```python
from build123d import *

# Parameters (mm, degrees)
F1_DEPTH = 1.524
F3_DEPTH = 2.54
F4_DEPTH = 3.81
F4_TAPER = 10
F5_W     = 16.791988407
F5_H     = 42.191988407
F6_DEPTH = 6.35


with BuildPart() as f1:
    # F0 (on Top) → F1 (new body)
    with BuildSketch(Plane.XY):
        with BuildLine():
            ThreePointArc((0, 3.175), (0.9299359697, 0.9299359697), (3.175, 0))
            Line((3.175, 0), (22.225, 0))
            ThreePointArc((22.225, 0), (24.4700640303, 0.9299359697), (25.4, 3.175))
            Line((25.4, 3.175), (25.4, 47.625))
            ThreePointArc((25.4, 47.625), (24.4700640303, 49.8700640303), (22.225, 50.8))
            Line((22.225, 50.8), (3.175, 50.8))
            ThreePointArc((3.175, 50.8), (0.9299359697, 49.8700640303), (0, 47.625))
            Line((0, 47.625), (0, 3.175))
        make_face()
    extrude(amount=F1_DEPTH)

    # F2 (on face) → F3 (join)
    with BuildSketch(Plane.XY.offset(1.524)):
        with BuildLine():
            Line((23.7998, 3.175), (23.7998, 47.625))
            ThreePointArc((23.7998, 47.625), (23.338551759, 48.738551759), (22.225, 49.1998))
            Line((22.225, 49.1998), (3.175, 49.1998))
            ThreePointArc((3.175, 49.1998), (2.061448241, 48.738551759), (1.6002, 47.625))
            Line((1.6002, 47.625), (1.6002, 3.175))
            ThreePointArc((1.6002, 3.175), (2.061448241, 2.061448241), (3.175, 1.6002))
            Line((3.175, 1.6002), (22.225, 1.6002))
            ThreePointArc((22.225, 1.6002), (23.338551759, 2.061448241), (23.7998, 3.175))
        make_face()
    extrude(amount=F3_DEPTH)

    # F3_face (on face) → F4 (join)
    with BuildSketch(Plane(origin=(12.7, 25.4, 4.064), x_dir=(1, 0, 0), z_dir=(0, 0, 1))):
        with BuildLine():
            ThreePointArc((9.525, -23.7998), (10.638551759, -23.338551759), (11.0998, -22.225))
            Line((11.0998, -22.225), (11.0998, 22.225))
            ThreePointArc((11.0998, 22.225), (10.638551759, 23.338551759), (9.525, 23.7998))
            Line((9.525, 23.7998), (-9.525, 23.7998))
            ThreePointArc((-9.525, 23.7998), (-10.638551759, 23.338551759), (-11.0998, 22.225))
            Line((-11.0998, 22.225), (-11.0998, -22.225))
            ThreePointArc((-11.0998, -22.225), (-10.638551759, -23.338551759), (-9.525, -23.7998))
            Line((-9.525, -23.7998), (9.525, -23.7998))
        make_face()
    extrude(amount=F4_DEPTH, taper=F4_TAPER)

    # F5 (on face) → F6 (cut)
    with BuildSketch(Plane.XY.offset(7.874)):
        with Locations((12.7, 25.4)):
            Rectangle(F5_W, F5_H)
    extrude(amount=-F6_DEPTH, mode=Mode.SUBTRACT)


solid = f1.part
```
The model under review builds one solid part; all positions refer to its coordinate system, in mm. A direction names the side the tool comes from. Round coordinates to 2 decimals unless told otherwise and drop trailing zeros. Loops run counter-clockwise (first coordinate to the right, second up) from the corner with the lowest first, then second, coordinate; pieces in that order, holes last. Notation, with made-up numbers: (26.5, 19) - (42.5, 19) arc R18 cw to (42.5, 23) - close; hole circle Ø3 at (24.5, 79.25). An arc over 180 degrees is marked (long way). Write each question's results on one line, items separated by ' | '. Start each with the question number.
Q1. Take a section at A-A on z = 3. Give the boundary of the cut face in (x, y) (3 decimals), plus the area to 3 significant figures.
Q2. Take a section at B-B on x = 7. Give the boundary of the cut face in (y, z).
Q3. Draft analysis for pull direction Y (two halves, no side actions). For faces 5 (the flat face through (21.096, 25, 5)), 6 (the flat face through (4.304, 25, 5)), 7 (the conical face through (2.293, 2.312, 5.996)), 8 (the flat face through (1.93, 25.09, 5.94)), state which applies: pulls with the +Y half, pulls with the -Y half, needs draft (parallel to the pull), parting line crosses it, or undercut.
Q4. Take a section at C-C on y = 6. Give the boundary of the cut face in (x, z).
Q5. Take a section at D-D on z = 6.25. Give the boundary of the cut face in (x, y) (3 decimals), plus the area to 3 significant figures.
Q6. Wall thickness on line 1 along X through (y, z) = (33, 2.75); line 2 along Y through (x, z) = (15.75, 1.75); line 3 along X through (y, z) = (20, 5.25): over which ranges is each line inside the solid? List them lowest first. Write a range as [from, to].
Q7. Insertion check: P1, Ø0.8, axis at x = 8, z = 2.5, coming from the +Y side; P2, Ø7.5, axis at x = 16, y = 24, coming from the +Z side; P3, Ø1.9, axis at x = 9, z = 5, coming from the -Y side. Each pin has a flat end and moves straight along its axis. Give the tip position at first contact, or say it passes through.
Q8. Tool access review of faces 1 (the flat face through (13, 49.2, 3)), 2 (the cylindrical face through (23.326, 2.049, 2.776)), 3 (the cylindrical face through (2.074, 48.751, 2.776)), 4 (the flat face through (13, 46.496, 5)): name each direction out of +Z, -Z, +X, -X, +Y, -Y from which nothing blocks a thin tool from reaching the whole face with its end or side.
Data:
1) outline: (1.6, 3.175) arc R1.575 ccw to (3.175, 1.6) - (22.225, 1.6) arc R1.575 ccw to (23.8, 3.175) - (23.8, 47.625) arc R1.575 ccw to (22.225, 49.2) - (3.175, 49.2) arc R1.575 ccw to (1.6, 47.625) - close; hole (4.304, 4.304) - (21.096, 4.304) - (21.096, 46.496) - (4.304, 46.496) - close | area: 346 mm²
2) outline: (0, 0) - (50.8, 0) - (50.8, 1.52) - (49.2, 1.52) - (49.2, 4.06) - (48.53, 7.87) - (46.5, 7.87) - (46.5, 1.52) - (4.3, 1.52) - (4.3, 7.87) - (2.27, 7.87) - (1.6, 4.06) - (1.6, 1.52) - (0, 1.52) - close
3) face 5: undercut | face 6: undercut | face 7: pulls with the -Y half | face 8: needs draft
4) outline: (0, 0) - (25.4, 0) - (25.4, 1.52) - (23.8, 1.52) - (23.8, 4.06) - (23.13, 7.87) - (21.1, 7.87) - (21.1, 1.52) - (4.3, 1.52) - (4.3, 7.87) - (2.27, 7.87) - (1.6, 4.06) - (1.6, 1.52) - (0, 1.52) - close
5) outline: (1.986, 3.175) arc R1.189 ccw to (3.175, 1.986) - (22.225, 1.986) arc R1.189 ccw to (23.414, 3.175) - (23.414, 47.625) arc R1.189 ccw to (22.225, 48.814) - (3.175, 48.814) arc R1.189 ccw to (1.986, 47.625) - close; hole (4.304, 4.304) - (21.096, 4.304) - (21.096, 46.496) - (4.304, 46.496) - close | area: 294 mm²
6) line 1: x = [1.6, 4.3], [21.1, 23.8] | line 2: y = [1.6, 4.3], [46.5, 49.2] | line 3: x = [1.81, 4.3], [21.1, 23.59]
7) P1: stops at y = 49.2 | P2: stops at z = 1.52 | P3: stops at y = 1.6
8) face 1: +Z, +X, -X, +Y | face 2: +Z, +X, -Y | face 3: +Z, -X, +Y | face 4: +Z
